```python
from build123d import *

# Parameters (mm, degrees)
ESQUISSE1_R        = 2.5
ESQUISSE1_R_2      = 5
BOSS_EXTRU_2_DEPTH = 3


with BuildPart() as part:
    # Esquisse1 → Boss.-Extru.2 (new body)
    with BuildSketch(Plane(origin=(0, 0, 0), x_dir=(1, 0, 0), z_dir=(0, 1, 0))):
        with BuildLine():
            ThreePointArc((0, -8), (1.852964218, -7.782449717), (3.605150215, -7.141630901))
            Line((3.605150215, -7.141630901), (10.5, -5.5))
            ThreePointArc((10.5, -5.5), (16, 0), (10.5, 5.5))
            Line((10.5, 5.5), (3.605150215, 7.141630901))
            ThreePointArc((3.605150215, 7.141630901), (0, 8), (-3.605150215, 7.141630901))
            Line((-3.605150215, 7.141630901), (-10.5, 5.5))
            ThreePointArc((-10.5, 5.5), (-16, 0), (-10.5, -5.5))
            Line((-10.5, -5.5), (0, -8))
        make_face()
        with Locations((-10.5, 0)):
            Circle(ESQUISSE1_R, mode=Mode.SUBTRACT)
        Circle(ESQUISSE1_R_2, mode=Mode.SUBTRACT)
        with Locations((10.5, 0)):
            Circle(ESQUISSE1_R, mode=Mode.SUBTRACT)
    extrude(amount=BOSS_EXTRU_2_DEPTH)


solid = part.part
```
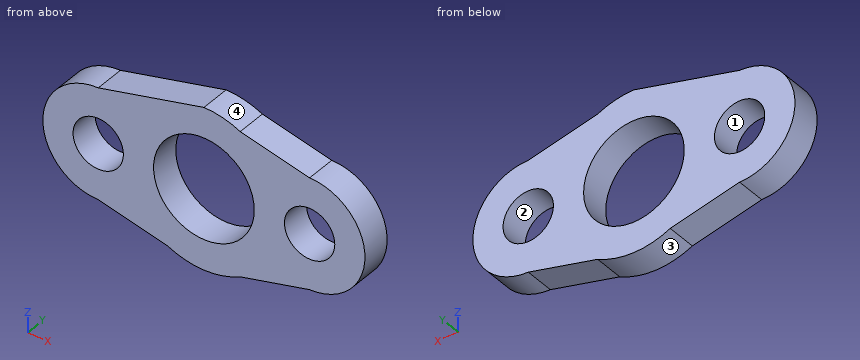
Can you work these out from the model? Positions are in its coordinate system, mm. Face numbers are marked on the shaded views. Give positions to 0.01 mm unless a question says otherwise; leave off trailing zeros. Order: outer loops, then holes, each group sorted by start corner. A loop starts at its lowest first (then second) coordinate and runs counter-clockwise, first axis right, second up. Notation, with made-up numbers: M 26.5,-10 L 76.5,-10 A12 cw 76.5,1 Z; hole C -13.5,60 d5. An arc over 180 degrees is marked long. Write item = value, one per line. Start each with the question number.
Q1. Will these pins go through, and if not, where does the flat tip stop? pin 1 Ø1 at (x, y) = (2, 2) entering from +Z; pin 2 Ø1.5 at (x, y) = (-12.5, 2) entering from +Z; pin 3 Ø1.5 at (x, y) = (9.5, 1) entering from -Z.
Q2. Suppose I cut it at D-D (z = 3.75). Write out the boundary of the cut face in (x, y), plus the area to 3 significant figures.
Q3. We'd pull the mould along X, two halves only. Please class the marked faces 1, 2, 3 and 4: pulls with the +X half, pulls with the -X half, needs draft (parallel to the pull), parting line crosses it, or undercut.
Q4. I need wall thicknesses on probe 1 along X at (y, z) = (2.1, 0); probe 2 along Z at (x, y) = (-10.5, 2.1); probe 3 along X at (y, z) = (2.45, 2.25). Which ranges of each line are inside material? Lowest first, please. Write a range as [from, to].
Q5. Suppose I cut it at C-C (x = -12). Write out the boundary of the cut face in (y, z).
Q6. Suppose I cut it at B-B (y = 1.4). Write out the boundary of the cut face in (x, z), plus the area to 3 significant figures.
Q7. Suppose I cut it at A-A (z = 0). Write out the boundary of the cut face in (x, y).
Check result:
q1.pin_1 = 7.86
q1.pin_2 = 5.36
q1.pin_3 = -5.92
q2.outline = M -14.52,0 L -3.31,0 L -3.31,3 L -14.52,3 Z; M 3.31,0 L 14.52,0 L 14.52,3 L 3.31,3 Z
q2.area = 67.3 mm2
q3.face_1 = undercut
q3.face_2 = undercut
q3.face_3 = parting line crosses it
q3.face_4 = pulls with the +X half
q4.probe_1 = [-16, -13], [-8, -5], [5, 8], [13, 16]
q4.probe_2 = [-5.5, -2.5], [2.5, 5.5]
q4.probe_3 = [-15.52, -11.59], [-9.41, -4.47], [4.47, 9.41], [11.59, 15.52]
q5.outline = M 0,-5.29 L 3,-5.29 L 3,-2 L 0,-2 Z; M 0,2 L 3,2 L 3,5.29 L 0,5.29 Z
q6.outline = M -10.5,-5.5 L -3.61,-7.14 A8 ccw 3.61,-7.14 L 10.5,-5.5 A5.5 ccw 10.5,5.5 L 3.61,7.14 A8 ccw 0,8 L -10.5,5.5 A5.5 ccw Z; hole C -10.5,0 d5; hole C 0,0 d10; hole C 10.5,0 d5
q6.area = 262 mm2
q7.outline = M -16,0 L -13,0 L -13,3 L -16,3 Z; M -8,0 L -5,0 L -5,3 L -8,3 Z; M 5,0 L 8,0 L 8,3 L 5,3 Z; M 13,0 L 16,0 L 16,3 L 13,3 Z
